```python
from build123d import *

# Parameters (mm, degrees)
F1_DEPTH = 2.5
F2_DEPTH = 10
F4_DEPTH = 2.5


with BuildPart() as f1:
    # F0 (on Front) → F1 (new body)
    with BuildSketch(Plane.XZ):
        Polygon((0, 20), (0, 0), (5, 0), (5, 2.5), (20, 2.5), (20, 14.6428571429), (12.5, 20), align=None)
        Polygon((30, 7.5), (20, 14.6428571429), (20, 2.5), (20, 0), (30, 0), align=None)
    extrude(amount=F1_DEPTH)

    # F0 (on Front) → F2 (join)
    with BuildSketch(Plane.XZ):
        Polygon((0, 20), (0, 0), (5, 0), (5, 2.5), (20, 2.5), (20, 14.6428571429), (12.5, 20), align=None)
    extrude(amount=F2_DEPTH)

    # F3 (on face) → F4 (join)
    with BuildSketch(Plane.XZ.offset(10)):
        Polygon((20, 2.5), (20, 14.6428571429), (12.5, 20), (0, 20), (0, 0), (5, 0), (5, 2.5), align=None)
        Polygon((30, 7.5), (20, 14.6428571429), (20, 2.5), (20, 0), (30, 0), align=None)
    extrude(amount=F4_DEPTH)


solid = f1.part
```
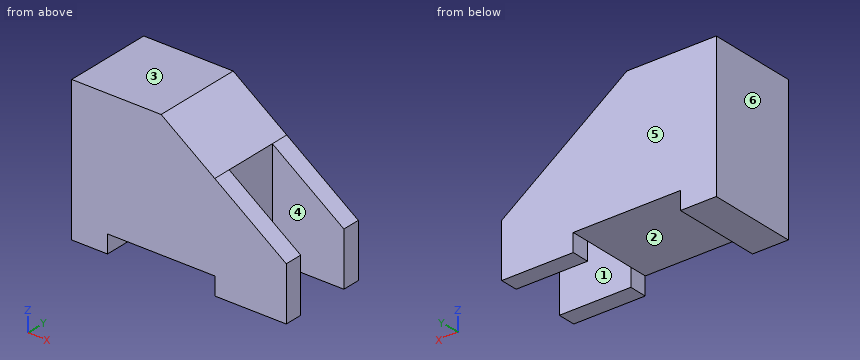
Verification items for the finished model (mm, model axes). Face numbers are marked on the shaded views. A direction names the side the tool comes from. Round coordinates to 2 decimals unless told otherwise and drop trailing zeros. Order: outer loops, then holes, each group sorted by start corner. A loop starts at its lowest first (then second) coordinate and runs counter-clockwise, first axis right, second up. Notation, with made-up numbers: (86.25, -5) -> (128.25, -5) arc R18 cw to (128.25, 21) -> close; hole circle Ø2 at (-11, 58.5). An arc over 180 degrees is marked (long way). Put each result on its own line as item: value. Start each with the question number.
(1) Section check C-C (y = -5.25). Enter the section's corners in (x, z), then the cut area to 3 significant figures.
(2) Section check D-D (z = 5). Enter the section's corners in (x, y), then the cut area to 3 significant figures.
(3) Material ranges on line 1 along Y through (x, z) = (20.75, 6.5); line 2 along X through (y, z) = (-1.5, 2); line 3 along X through (y, z) = (-2.75, 6), recorded low to high.
(4) Depth check by flat-ended pin: pin 1 Ø1.2 at (y, z) = (-7, 1) entering from +X; pin 2 Ø1 at (x, y) = (16.5, -1.5) entering from +Z. Enter the tip coordinate at first touch or a pass-through.
(5) Tool access check on the marked faces 1, 2 and 3. Record the directions out of +Z, -Z, +X, -X, +Y, -Y that give a thin tool (end or side, any length) a straight path to the whole face; none if there is none.
(6) Section check A-A (x = 23). Enter the section's corners in (y, z).
(7) Draft check along Y on the marked faces 4, 5 and 6. Enter one of: +Y half, -Y half, draft (parallel to the pull), parting line (faces both ways), or undercut.
(8) Section check B-B (z = 13). Enter the section's corners in (x, y).
Completed:
1. outline: (0, 0) -> (5, 0) -> (5, 2.5) -> (20, 2.5) -> (20, 14.64) -> (12.5, 20) -> (0, 20) -> close
1. area: 342 mm2
2. outline: (0, -12.5) -> (30, -12.5) -> (30, -10) -> (20, -10) -> (20, -2.5) -> (30, -2.5) -> (30, 0) -> (0, 0) -> close
2. area: 300 mm2
3. line 1: y = -12.5 to -10, -2.5 to 0
3. line 2: x = 0 to 5, 20 to 30
3. line 3: x = 0 to 20
4. pin 1: stops at x = 5
4. pin 2: stops at z = 17.5
5. face 1: +Z, -Z, +X
5. face 2: -Z, +Y, -Y
5. face 3: +Z, +X, -X, +Y, -Y
6. outline: (-12.5, 0) -> (-10, 0) -> (-10, 12.5) -> (-12.5, 12.5) -> close; (-2.5, 0) -> (0, 0) -> (0, 12.5) -> (-2.5, 12.5) -> close
7. face 4: undercut
7. face 5: +Y half
7. face 6: draft
8. outline: (0, -12.5) -> (22.3, -12.5) -> (22.3, -10) -> (20, -10) -> (20, -2.5) -> (22.3, -2.5) -> (22.3, 0) -> (0, 0) -> close
